Geometry check sheet. Reference: drawing and pictorial views, mm from the part's lowest x, y, z. Give positions to 0.01 mm unless a question says otherwise; leave off trailing zeros. Loops run counter-clockwise (first coordinate to the right, second up) from the corner with the lowest first, then second, coordinate; pieces in that order, holes last. Notation, with made-up numbers: (83.25, 2.25) - (97.25, 2.25) arc R19 cw to (97.25, 33.25) - close; hole circle Ø9 at (-25.75, -23.75). An arc over 180 degrees is marked (long way). Answer in a Markdown table with one row per item. Add a question column.
(1) Sectioned sample at A-A on z = 6.35. Enter the section's corners in (x, y) (1 decimal).
(2) Sectioned sample at B-B on x = 5.5. Enter the section's corners in (y, z) (1 decimal), then the cut area to 3 significant figures.
(3) Sectioned sample at D-D on y = 12.5. State how many separate pieces and enclosed holes the cut face has.
(4) Sectioned sample at C-C on z = 55. Enter the section's corners in (x, y) (1 decimal).
(5) Thickness scan on L1, parallel to Z at x = 4.75, y = 5 (1 decimal); L2, parallel to Z at x = 4, y = 18.5 (1 decimal). Record the ranges inside material, lowest first.
(6) Go/stop test with flat-tipped pins: P1, Ø3, axis at x = 4.76, z = 6.35, coming from the -Y side; P2, Ø4, axis at x = 7, y = 12, coming from the -Z side. Record where each tip stops, or that it passes through.
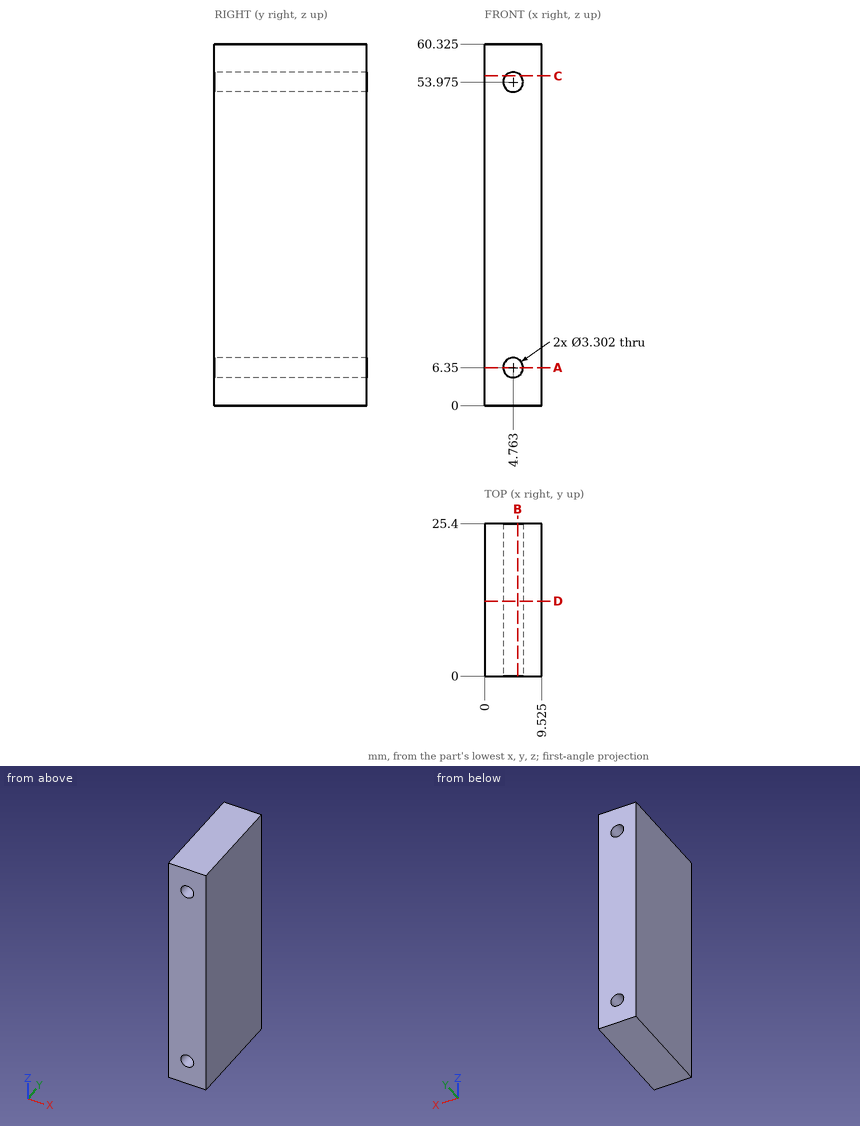
Reply:
| question | item | result |
|---|---|---|
| 1 | outline | (0, 0) - (3.1, 0) - (3.1, 25.4) - (0, 25.4) - close; (6.4, 0) - (9.5, 0) - (9.5, 25.4) - (6.4, 25.4) - close |
| 2 | outline | (0, 0) - (25.4, 0) - (25.4, 4.9) - (0, 4.9) - close; (0, 7.8) - (25.4, 7.8) - (25.4, 52.5) - (0, 52.5) - close; (0, 55.5) - (25.4, 55.5) - (25.4, 60.3) - (0, 60.3) - close |
| 2 | area | 1,380 mm^2 |
| 3 | separate pieces | 1 |
| 3 | enclosed holes | 2 |
| 4 | outline | (0, 0) - (3.5, 0) - (3.5, 25.4) - (0, 25.4) - close; (6.1, 0) - (9.5, 0) - (9.5, 25.4) - (6.1, 25.4) - close |
| 5 | L1 | 0 to 4.7, 8 to 52.3, 55.6 to 60.3 |
| 5 | L2 | 0 to 4.9, 7.8 to 52.5, 55.4 to 60.3 |
| 6 | P1 | through |
| 6 | P2 | z = 0 |
